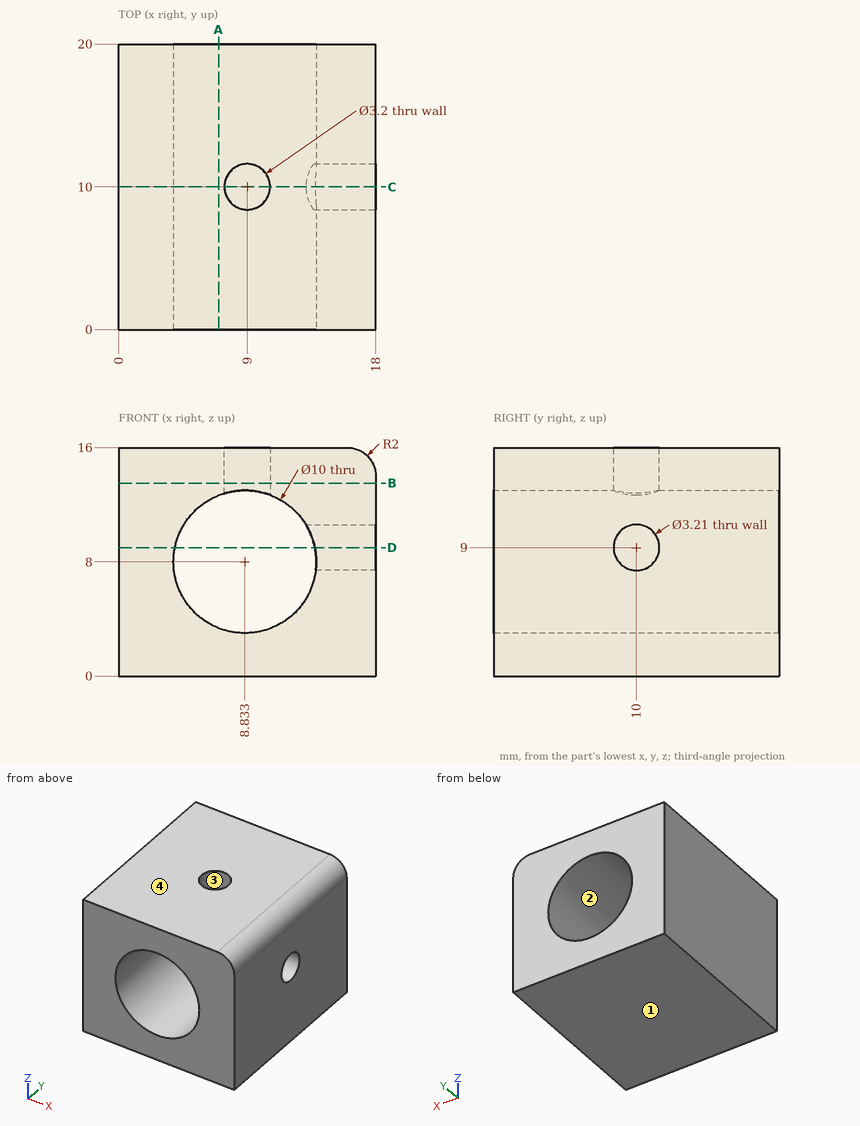
Drawing for the job (mm, zero at the part's lowest x, y, z). Round coordinates to 2 decimals unless told otherwise and drop trailing zeros. Write each loop counter-clockwise with the first axis right and the second up, starting at its lowest first coordinate (ties: lowest second). Pieces come first, ordered by that corner, then holes. Notation, with made-up numbers: M 44,46 L 101,46 A14 ccw 101,63 Z; hole C 66.25,-8.75 d1. An arc over 180 degrees is marked long. Answer as a JSON object with one key per item and string values. Group by question number.
(1) Mould opens along Z. For the marked faces 1, 2, 3 and 4 say: pulls with the +Z half, pulls with the -Z half, needs draft (parallel to the pull), parting line crosses it, or undercut.
(2) Drill centre lines: L1, parallel to Z at x = 8.75, y = 4.25; L2, parallel to Y at x = 9, z = 14.9; L3, parallel to X at y = 5.75, z = 8. Where is each one in solid material? Low to high.
(3) Cut at B-B (z = 13.5). Give the cut face in (x, y).
(4) Cut at A-A (x = 7). Give the cut face in (y, z).
(5) Cut at C-C (y = 10). Give the cut face in (x, z) (1 decimal), and give its area (3 significant figures).
(6) Cut at D-D (z = 9). Give the cut face in (x, y) (1 decimal), and give its area (3 significant figures).
Responses:
{
 "1": {"face 1": "pulls with the -Z half", "face 2": "undercut", "face 3": "needs draft", "face 4": "pulls with the +Z half"},
 "2": {"L1": "z = 0 to 3, 13 to 16", "L2": "y = 0 to 8.4, 11.6 to 20", "L3": "x = 0 to 3.83, 13.83 to 18"},
 "3": {"outline": "M 0,0 L 18,0 L 18,20 L 0,20 Z; hole C 9,10 d3.2"},
 "4": {"outline": "M 0,0 L 20,0 L 20,3.35 L 0,3.35 Z; M 0,12.65 L 20,12.65 L 20,16 L 0,16 Z"},
 "5": {"outline": "M 0,0 L 18,0 L 18,7.4 L 13.8,7.4 A5 cw long 7.4,12.8 L 7.4,16 L 0,16 Z; M 10.6,12.7 A5 cw 13.1,10.6 L 18,10.6 L 18,14 A2 ccw 16,16 L 10.6,16 Z", "area": "185 mm2"},
 "6": {"outline": "M 0,0 L 3.9,0 L 3.9,20 L 0,20 Z; M 13.7,0 L 18,0 L 18,8.4 L 13.7,8.4 Z; M 13.7,11.6 L 18,11.6 L 18,20 L 13.7,20 Z", "area": "150 mm2"}
}
